Could you check a few things on this model? Use its own coordinates, in mm. A direction names the side the tool comes from. Coordinates: 2 decimals unless noted, no trailing zeros. Loops run counter-clockwise (first coordinate to the right, second up) from the corner with the lowest first, then second, coordinate; pieces in that order, holes last. Notation, with made-up numbers: (33.25, 67) - (82.25, 67) arc R15 ccw to (82.25, 75) - close; hole circle Ø4 at (80.25, -12). An arc over 180 degrees is marked (long way). One line per item, written item: value. Start each with the question number.
(1) If we section it at A-A on x = -25: Write out the boundary of the cut face in (y, z) (3 decimals).
(2) On a 3-axis mill with a long thin cutter (end or side, diameter ignored), from which of +Z, -Z, +X, -X, +Y, -Y can I reach the whole of each face in a straight line? I mean faces 1 (the face through (-351.755, -9.824, -2.182)), 2 (the face through (253.86, -12.15, -2.7)), 3 (the face through (-365.281, -6.76, -8.817)). Say none if no direction works.
(3) I'm going to push flat-ended pins straight in: P1, Ø1, axis at x = 19.5, z = -4.5, coming from the -Y side; P2, Ø6, axis at x = -93, z = 8.5, coming from the +Y side; P3, Ø10, axis at x = -148.5, z = -3, coming from the +Y side (3 decimals). Where does each tip first touch, or does it pass through?
(4) If I drill on line 1 along X through (y, z) = (7, 7); line 2 along Z through (x, y) = (14, 0.5) (3 decimals); line 3 along Y through (x, z) = (-324, -5.25), over which ranges is the centre line in solid material (lowest first)? Write a range as from..to.
(5) If we mould it in two halves opening along X, with no side actions, what happens to faces 4 (the face through (11.47, -4.79, 11.54)), 5 (the face through (123.674, 2.861, 9.085)), 6 (the face through (0, 13, 0))? For each: pulls with the +X half, pulls with the -X half, needs draft (parallel to the pull), parting line crosses it, or undercut.
```python
from build123d import *

# Parameters (mm, degrees)
F4_R = 0.25
F5_R = 5
F6_R = 5


# Not quite as in the source:
# - a fillet or chamfer that OpenCascade refuses, or shapes differently, is made with other operations: its cross-section is extruded or revolved along the edge and cut away or added


with BuildPart() as f1:
    # F0 (on Front) → F1 (revolve)
    with BuildSketch(Plane.XZ):
        with BuildLine():
            Line((-2, 9.525), (-350.6009565311, 9.525))
            Line((-350.6009565311, 9.525), (-354, 11.11))
            Line((-354, 11.11), (-376.25, 11.11))
            Line((-376.25, 11.11), (-385, 8))
            Line((-385, 8), (-385, 0))
            Line((-385, 0), (297.49, 0))
            Line((297.49, 0), (297.49, 8.1239745962))
            Line((297.49, 8.1239745962), (295.99, 8.99))
            Line((295.99, 8.99), (285.0470138467, 8.99))
            ThreePointArc((285.0470138467, 8.99), (283.6876657265, 8.797737003), (282.5958183581, 9.63))
            Line((282.5958183581, 9.63), (280.97, 12.446))
            Line((280.97, 12.446), (227.5, 12.446))
            Line((227.5, 12.446), (224.579, 9.525))
            Line((224.579, 9.525), (23, 9.525))
            Line((23, 9.525), (23, 12.495))
            Line((23, 12.495), (0, 12.495))
            Line((0, 12.495), (0, 14.35))
            Line((0, 14.35), (-2, 14.35))
            Line((-2, 14.35), (-2, 9.525))
        make_face()
    revolve(axis=Axis((-43.755, 0, 0), (-1, 0, 0)))

    # F2: fillet of radius 8 on 1 edges, made by hand

    # F2_s1 → F2_t2 (revolve)
    with BuildSketch(Plane.XZ):
        with BuildLine():
            ThreePointArc((-2, 14.35), (-4.9498048155, 10.8391941398), (-9.3429813428, 9.525))
            Line((-9.3429813428, 9.525), (-2, 9.525))
            Line((-2, 9.525), (-2, 14.35))
        make_face()
    revolve(axis=Axis((-2, 0, 0), (-1, 0, 0)))

    # F3: fillet of radius 5 on 1 edges, made by hand

    # F3_s1 → F3_t2 (revolve)
    with BuildSketch(Plane.XZ):
        with BuildLine():
            ThreePointArc((27.5693653826, 9.525), (24.8444800639, 10.3327452367), (23, 12.495))
            Line((23, 12.495), (23, 9.525))
            Line((23, 9.525), (27.5693653826, 9.525))
        make_face()
    revolve(axis=Axis((23, 0, 0), (-1, 0, 0)))

    # F4
    f4_edges = [f1.edges().sort_by_distance(p)[0] for p in [
        (0, 0, -12.495),
    ]]
    fillet(f4_edges, radius=F4_R)

    # F5
    f5_edges = [f1.edges().sort_by_distance(p)[0] for p in [
        (-350.600957, 0, -9.525),
    ]]
    fillet(f5_edges, radius=F5_R)

    # F6
    f6_edges = [f1.edges().sort_by_distance(p)[0] for p in [
        (224.579, 0, -9.525),
    ]]
    fillet(f6_edges, radius=F6_R)


solid = f1.part
```
Values:
1. outline: circle Ø19.05 at (0, 0)
2. face 1: none
2. face 2: +X
2. face 3: -X
3. P1: stops at y = -11.84
3. P2: stops at y = 7.78
3. P3: stops at y = 9.525
4. line 1: x = -379.66..-351.39, -6.92..25.67, 224.41..282.44
4. line 2: z = -12.485..12.485
4. line 3: y = -7.95..7.95
5. face 4: needs draft
5. face 5: undercut
5. face 6: pulls with the +X half
